from build123d import *

# Parameters (mm, degrees)
F0_R     = 2
F0_R_2   = 1.5
F1_DEPTH = 1


with BuildPart() as f1:
    # F0 (on Top) → F1 (new body)
    with BuildSketch(Plane.XY):
        Polygon((36.9193002582, 80.5819368362), (-38.0806997418, 80.5819368362), (-38.0806997418, 20.6310992315), (-38.0806997418, 15.5746781826), (-38.0806997418, 8.1310992315), (-38.0806997418, 0.5819368409), (-38.0806997418, -6.8689007685), (-38.0806997418, -14.4253218174), (-38.0806997418, -19.3689007685), (-38.0806997418, -79.4180631638), (36.9193002582, -79.4180631638), (36.9193002582, -19.3689007685), (36.9193002582, -14.4253218174), (36.9193002582, -6.8689007685), (36.9193002582, 0.5819368362), (36.9193002582, 8.1310992315), (36.9193002582, 15.5746781826), (36.9193002582, 20.6310992315), align=None)
        with Locations((-35.0806997418, -76.3197383732)):
            Circle(F0_R, mode=Mode.SUBTRACT)
        Polygon((-33.3470307291, -54.2283378169), (-8.3470307291, -54.2283378169), (-8.3470307291, -74.2283378169), align=None, mode=Mode.SUBTRACT)
        Polygon((-33.3470307291, -48.6858622357), (-33.3470307291, -28.6858622357), (-8.3470307291, -48.6858622357), align=None, mode=Mode.SUBTRACT)
        Polygon((-33.3470307291, -20.2283378169), (-8.3470307291, -20.2283378169), (-8.3470307291, -40.2283378169), align=None, mode=Mode.SUBTRACT)
        Polygon((6.6529692709, -74.2283378169), (6.6529692709, -54.2283378169), (31.6529692709, -54.2283378169), align=None, mode=Mode.SUBTRACT)
        with Locations((33.9193002582, -76.3197383732)):
            Circle(F0_R, mode=Mode.SUBTRACT)
        Polygon((31.6529692709, -48.6858622357), (6.6529692709, -48.6858622357), (31.6529692709, -28.6858622357), align=None, mode=Mode.SUBTRACT)
        Polygon((6.6529692709, -40.2283378169), (6.6529692709, -20.2283378169), (31.6529692709, -20.2283378169), align=None, mode=Mode.SUBTRACT)
        with BuildLine():
            ThreePointArc((-35.0806997418, 0.5819368362), (-36.5806997442, -0.9180631638), (-38.0806997418, 0.5819368409))
            ThreePointArc((-38.0806997418, 0.5819368409), (-36.5806997395, 2.0819368362), (-35.0806997418, 0.5819368362))
        make_face(mode=Mode.SUBTRACT)
        Polygon((-8.3470307291, 41.7716621831), (-8.3470307291, 21.7716621831), (-33.3470307291, 21.7716621831), align=None, mode=Mode.SUBTRACT)
        Polygon((-8.3470307291, 50.2291866019), (-33.3470307291, 30.2291866019), (-33.3470307291, 50.2291866019), align=None, mode=Mode.SUBTRACT)
        with Locations((-35.0806997418, 77.5819368362)):
            Circle(F0_R, mode=Mode.SUBTRACT)
        Polygon((-8.3470307291, 55.7716621831), (-33.3470307291, 55.7716621831), (-8.3470307291, 75.7716621831), align=None, mode=Mode.SUBTRACT)
        Polygon((31.6529692709, 21.7716621831), (6.6529692709, 21.7716621831), (6.6529692709, 41.7716621831), align=None, mode=Mode.SUBTRACT)
        Polygon((31.6529692709, 50.2291866019), (31.6529692709, 30.2291866019), (6.6529692709, 50.2291866019), align=None, mode=Mode.SUBTRACT)
        with Locations((35.4193002582, 0.5819368362)):
            Circle(F0_R_2, mode=Mode.SUBTRACT)
        Polygon((31.6529692709, 55.7716621831), (6.6529692709, 55.7716621831), (6.6529692709, 75.7716621831), align=None, mode=Mode.SUBTRACT)
        with Locations((33.9193002582, 77.5819368362)):
            Circle(F0_R, mode=Mode.SUBTRACT)
        Polygon((38.9193002582, 8.1310992315), (36.9193002582, 8.1310992315), (36.9193002582, 0.5819368362), (36.9193002582, -6.8689007685), (38.9193002582, -6.8689007685), (38.9193002582, -4.3689007685), (38.9193002582, 5.6310992315), align=None)
        Polygon((-38.0806997418, 0.5819368409), (-38.0806997418, 8.1310992315), (-40.0806997418, 8.1310992315), (-40.0806997418, 5.6310992315), (-40.0806997418, -4.3689007685), (-40.0806997418, -6.8689007685), (-38.0806997418, -6.8689007685), align=None)
    extrude(amount=F1_DEPTH)


solid = f1.part
Design review of the part built by this model. Coordinates are the model's own, in mm. A direction names the side the tool comes from. Round coordinates to 2 decimals unless told otherwise and drop trailing zeros. Loops run counter-clockwise (first coordinate to the right, second up) from the corner with the lowest first, then second, coordinate; pieces in that order, holes last. Notation, with made-up numbers: M 33.25,-25 L 64.25,-25 A31 ccw 64.25,8 Z; hole C 45,1.25 d6. An arc over 180 degrees is marked long. Answer as a JSON object with one key per item and string values.
Item 1: Clearance check with flat-ended pins moving along their axes: P1, Ø0.5, axis at x = -39, z = 0.5, coming from the -Y side; P2, Ø3, axis at x = 33.92, y = 77.58, coming from the -Z side; P3, Ø0.5, axis at x = 37.5, z = 0.5, coming from the +Y side. State where each tip first meets the part, or that it passes through.
Answer sheet:
{"P1": "stops at y = -6.87", "P2": "passes through", "P3": "stops at y = 8.13"}
Item 2: We need section C-C on y = 52. Give the boundary of the cut face in (x, z), and give its area (3 significant figures).
Answer sheet:
{"outline": "M -38.08,0 L 36.92,0 L 36.92,1 L -38.08,1 Z", "area": "75.0 mm^2"}
Item 3: Machinability: for faces 1 (the flat face through (-20.67, -64.37, 0.49)), 2 (the flat face through (-1, 2, 0)), which of the approach directions +Z, -Z, +X, -X, +Y, -Y give a long, thin tool a straight path to every point of the face, cutting with its end or side? Answer none if there is none.
Answer sheet:
{"face 1": "+Z, -Z", "face 2": "-Z, +X, -X, +Y, -Y"}
Item 4: Wall thickness on L1, parallel to X at y = 0.5, z = 0.7; L2, parallel to X at y = -29, z = 0.85; L3, parallel to X at y = 71.5, z = 0.15: over which ranges is each line inside the solid? List them lowest first. Write a range as from..to.
Answer sheet:
{"L1": "x = -40.08..-38.08, -35.08..33.92, 36.92..38.92", "L2": "x = -38.08..-33.35, -32.95..-22.38, -8.35..6.65, 20.69..31.26, 31.65..36.92", "L3": "x = -38.08..-13.69, -8.35..6.65, 11.99..36.92"}
Item 5: We need section B-B on y = -44. Give the boundary of the cut face in (x, z), and give its area (3 significant figures).
Answer sheet:
{"outline": "M -38.08,0 L -33.35,0 L -33.35,1 L -38.08,1 Z; M -14.2,0 L 12.51,0 L 12.51,1 L -14.2,1 Z; M 31.65,0 L 36.92,0 L 36.92,1 L 31.65,1 Z", "area": "36.7 mm^2"}
Item 6: We need section A-A on x = -14.5. Give the boundary of the cut face in (y, z), and give its area (3 significant figures).
Answer sheet:
{"outline": "M -79.42,0 L -69.31,0 L -69.31,1 L -79.42,1 Z; M -54.23,0 L -48.69,0 L -48.69,1 L -54.23,1 Z; M -43.76,0 L -35.31,0 L -35.31,1 L -43.76,1 Z; M -20.23,0 L 21.77,0 L 21.77,1 L -20.23,1 Z; M 36.85,0 L 45.31,0 L 45.31,1 L 36.85,1 Z; M 50.23,0 L 55.77,0 L 55.77,1 L 50.23,1 Z; M 70.85,0 L 80.58,0 L 80.58,1 L 70.85,1 Z", "area": "89.8 mm^2"}
Item 7: We need section D-D on x = -30. Give the boundary of the cut face in (y, z), and give its area (3 significant figures).
Answer sheet:
{"outline": "M -79.42,0 L -56.91,0 L -56.91,1 L -79.42,1 Z; M -54.23,0 L -48.69,0 L -48.69,1 L -54.23,1 Z; M -31.36,0 L -22.91,0 L -22.91,1 L -31.36,1 Z; M -20.23,0 L 21.77,0 L 21.77,1 L -20.23,1 Z; M 24.45,0 L 32.91,0 L 32.91,1 L 24.45,1 Z; M 50.23,0 L 55.77,0 L 55.77,1 L 50.23,1 Z; M 58.45,0 L 80.58,0 L 80.58,1 L 58.45,1 Z", "area": "115 mm^2"}
